```python
from build123d import *

# Parameters (mm, degrees)
F0_W     = 90
F0_H     = 90
F1_DEPTH = 5
F3_DEPTH = 2
F4_R     = 25


with BuildPart() as f1:
    # F0 (on Top) → F1 (new body)
    with BuildSketch(Plane.XY):
        Rectangle(F0_W, F0_H)
    extrude(amount=F1_DEPTH)

    # F2 (on face) → F3 (join)
    with BuildSketch(Plane.XY.offset(5)):
        with BuildLine():
            Line((14, 41), (-4, 41))
            ThreePointArc((-4, 41), (-30.162951, 30.162951), (-41, 4))
            Line((-41, 4), (-41, -9))
            ThreePointArc((-41, -9), (-31.627417, -31.627417), (-9, -41))
            Line((-9, -41), (-1, -41))
            ThreePointArc((-1, -41), (28.698485, -28.698485), (41, 1))
            Line((41, 1), (41, 14))
            ThreePointArc((41, 14), (33.091883, 33.091883), (14, 41))
        make_face()
        with BuildLine():
            ThreePointArc((-29, 5), (-21.970563, 21.970563), (-5, 29))
            Line((-5, 29), (15, 29))
            ThreePointArc((15, 29), (24.899495, 24.899495), (29, 15))
            Line((29, 15), (29, -10))
            ThreePointArc((29, -10), (23.435029, -23.435029), (10, -29))
            Line((10, -29), (-20, -29))
            ThreePointArc((-20, -29), (-26.363961, -26.363961), (-29, -20))
            Line((-29, -20), (-29, 5))
        make_face(mode=Mode.SUBTRACT)
    extrude(amount=F3_DEPTH)

    # F4
    f4_edges = [f1.edges().sort_by_distance(p)[0] for p in [
        (-45, -45, 2.5),
        (45, -45, 2.5),
        (45, 45, 2.5),
        (-45, 45, 2.5),
    ]]
    fillet(f4_edges, radius=F4_R)


solid = f1.part
```
Model file for the job. Use its own axes, mm. A direction names the side the tool comes from. Coordinates: 2 decimals unless noted, no trailing zeros. Write each loop counter-clockwise with the first axis right and the second up, starting at its lowest first coordinate (ties: lowest second). Pieces come first, ordered by that corner, then holes. Notation, with made-up numbers: (60.5, 34) - (70.5, 34) arc R17 cw to (70.5, 43) - close; hole circle Ø6 at (80.25, -16). An arc over 180 degrees is marked (long way). One line per item, written item: value. Start each with the question number.
1. Slice it at C-C (x = -22). Write the cut outline in (y, z), plus the area to 3 significant figures.
2. Tool access for faces 5 (the cylindrical face through (23.58, -23.29, 5.99)), 6 (the flat face through (-41, -2, 6)), 7 (the cylindrical face through (28.37, -29.023, 5.986)), 8 (the cylindrical face through (-29.87, 30.45, 5.99)): list every direction of +Z, -Z, +X, -X, +Y, -Y with a clear straight run to the whole face (end or side of a thin tool).
3. Slice it at D-D (y = -14). Write the cut outline in (x, z), plus the area to 3 significant figures.
4. Probe line 1 (X direction, y = 1, z = 6.75); line 2 (Z direction, x = -11.5, y = 1). List the from-to ranges inside material, lowest first. Write a range as from..to.
5. Flat gauge pins, fed straight in: pin 1 (17.5 mm diameter, centred on x = -13, y = -4.5, fed in from +Z); pin 2 (0.6 mm diameter, centred on x = 3, z = 6, fed in from +Y); pin 3 (1 mm diameter, centred on x = -34, z = 4, fed in from -Y). Where does each tip first touch, or does it go through?
6. Slice it at A-A (z = 1.5). Write the cut outline in (x, y).
7. Mould opens along Y. For faces 1 (the flat face through (5, 29, 6)), 2 (the flat face through (0, -45, 2)), 3 (the flat face through (10, -40, 5)), 4 (the cylindrical face through (33.3, 32.88, 5.99)) say: released by +Y, released by -Y, zero draft, split by the parting line, or undercut.
8. Slice it at B-B (y = -30.5). Write the cut outline in (x, z), plus the area to 3 significant figures.
Answers below:
1. outline: (-44.92, 0) - (44.92, 0) - (44.92, 5) - (36.33, 5) - (36.33, 7) - (21.94, 7) - (21.94, 5) - (-28.77, 5) - (-28.77, 7) - (-38.24, 7) - (-38.24, 5) - (-44.92, 5) - close
1. area: 497 mm^2
2. face 5: +Z
2. face 6: +Z, -X, +Y, -Y
2. face 7: +Z, +X, -Y
2. face 8: +Z, -X, +Y
3. outline: (-45, 0) - (45, 0) - (45, 5) - (38.23, 5) - (38.23, 7) - (28.57, 7) - (28.57, 5) - (-29, 5) - (-29, 7) - (-40.61, 7) - (-40.61, 5) - (-45, 5) - close
3. area: 493 mm^2
4. line 1: x = -41..-29, 29..41
4. line 2: z = 0..5
5. pin 1: stops at z = 5
5. pin 2: stops at y = 41
5. pin 3: stops at y = -41.04
6. outline: (-45, -20) arc R25 ccw to (-20, -45) - (20, -45) arc R25 ccw to (45, -20) - (45, 20) arc R25 ccw to (20, 45) - (-20, 45) arc R25 ccw to (-45, 20) - close
7. face 1: undercut
7. face 2: released by -Y
7. face 3: zero draft
7. face 4: released by +Y
8. outline: (-42.69, 0) - (42.69, 0) - (42.69, 5) - (26.78, 5) - (26.78, 7) - (-32.7, 7) - (-32.7, 5) - (-42.69, 5) - close
8. area: 546 mm^2
